Drawing for the job (mm, zero at the part's lowest x, y, z). Coordinates: 2 decimals unless noted, no trailing zeros. Order: outer loops, then holes, each group sorted by start corner. A loop starts at its lowest first (then second) coordinate and runs counter-clockwise, first axis right, second up. Notation, with made-up numbers: (3, 84) - (59, 84) arc R7 ccw to (59, 95) - close; hole circle Ø11 at (-32, 89.5). An arc over 180 degrees is marked (long way). Answer as CSV lines item,"result". Start each with the question number.
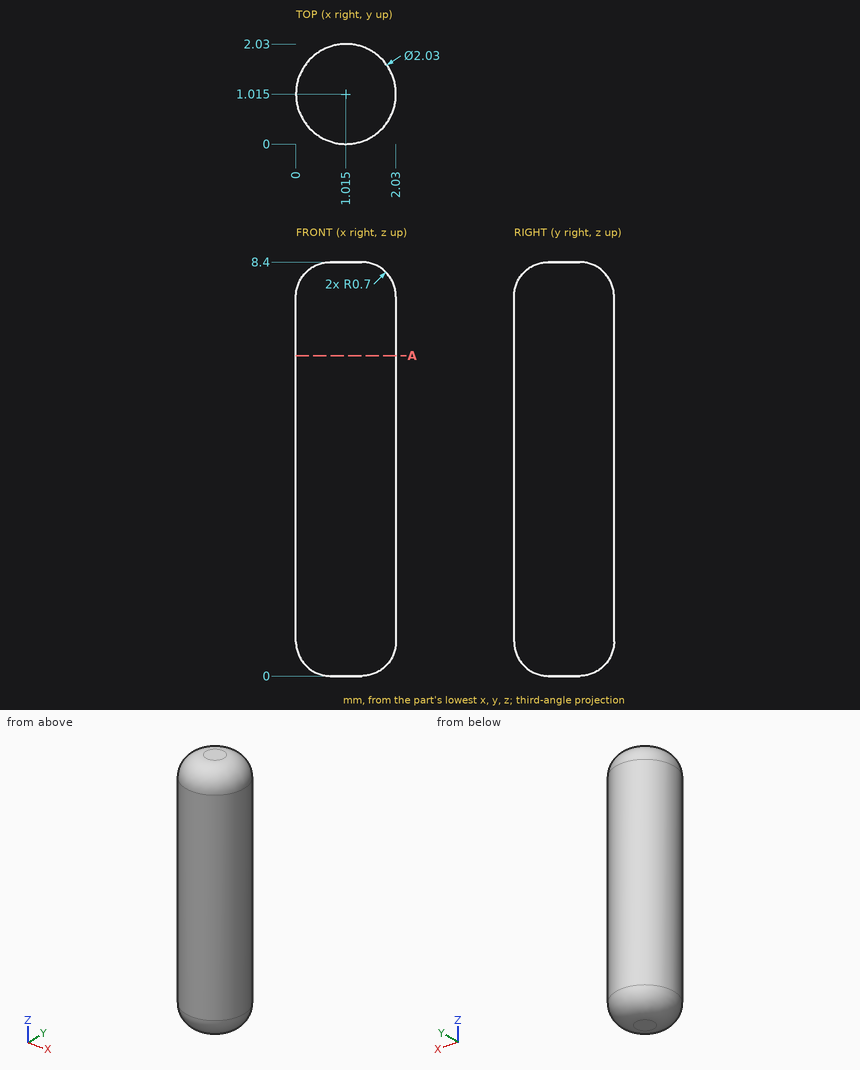
(1) Probe L1, parallel to Y at x = 0.55, z = 2.5; L2, parallel to X at y = 1.6, z = 4.5; L3, parallel to Z at x = 0.1, y = 0.95. List the from-to ranges inside material, lowest first. Write a range as [from, to].
(2) Band-saw the part on A-A on z = 6.5. List the corners of the cut face in (x, y) (3 decimals), plus the area to 3 significant figures.
(3) Drop a flat-ended pin along its axis: pin 1 Ø1 at (x, y) = (2, 0.5) entering from -Z. Give the stop position or say it passes through.
Filled in:
1,L1,"y = [0.11, 1.92]"
1,L2,"x = [0.19, 1.84]"
1,L3,"z = [0.34, 8.06]"
2,outline,"circle Ø2.03 at (1.015, 1.015)"
2,area,"3.24 mm^2"
3,pin 1,"stops at z = 0.07"
